For this review, take the finished solid that the model builds, in its own axes (mm). A direction names the side the tool comes from. Round coordinates to 2 decimals unless told otherwise and drop trailing zeros. Loops run counter-clockwise (first coordinate to the right, second up) from the corner with the lowest first, then second, coordinate; pieces in that order, holes last.
1. Draft analysis for pull direction Z (two halves, no side actions). For faces 1 (the cylindrical face through (2.958, 2.281, -123.594)), 2 (the flat face through (0, 91, -62)), 3 (the cylindrical face through (2.96, 44.25, -111.05)), state which applies: released by +Z, released by -Z, zero draft, split by the parting line, or undercut.
2. Tool access review of faces 4 (the cylindrical face through (2.96, 123.75, -38.91)), 5 (the flat face through (6, 91, -62)): name each direction out of +Z, -Z, +X, -X, +Y, -Y from which nothing blocks a thin tool from reaching the whole face with its end or side.
3. Consider section A-A on z = -111. State the section outline as (x, y) points, then the cut area to 3 significant figures.
4. Consider section B-B on y = 162.5. State the section outline as (x, z) points, then the cut area to 3 significant figures.
5. To check wall thickness, follow line 1 along Z through (x, y) = (5.35, 162); line 2 along Y through (x, z) = (4.45, -109); line 3 along Z through (x, y) = (3.2, 167.5). State the ranges of each line that lie inside material, in increasing order.
6. Consider section C-C on x = 1.5. State how many separate pieces and enclosed holes the cut face has, then the cut area to 3 significant figures.
from build123d import *

# Parameters (mm, degrees)
EXTRUDE_2_DEPTH          = 6
CUT_EXTRUDE_1_DEPTH      = 7
CUT_EXTRUDE_1_DEPTH_BACK = 1


with BuildPart() as part:
    # 草图1 → 凸台-拉伸2 (new body)
    with BuildSketch(Plane(origin=(0, 0, 0), x_dir=(0, 0, -1), z_dir=(1, 0, 0))):
        with BuildLine():
            Line((8, 0), (118, 0))
            ThreePointArc((118, 0), (123.656854249, 2.343145751), (126, 8))
            Line((126, 8), (126, 171.5))
            ThreePointArc((126, 171.5), (123.656854249, 177.156854249), (118, 179.5))
            Line((118, 179.5), (8, 179.5))
            ThreePointArc((8, 179.5), (2.343145751, 177.156854249), (0, 171.5))
            Line((0, 171.5), (0, 8))
            ThreePointArc((0, 8), (2.343145751, 2.343145751), (8, 0))
        make_face()
        with BuildLine():
            Line((12.75, 10), (12.75, 8))
            ThreePointArc((12.75, 8), (15, 5.75), (17.25, 8))
            Line((17.25, 8), (17.25, 10))
            ThreePointArc((17.25, 10), (15, 12.25), (12.75, 10))
        make_face(mode=Mode.SUBTRACT)
        with BuildLine():
            Line((12.75, 42), (12.75, 40))
            ThreePointArc((12.75, 40), (15, 37.75), (17.25, 40))
            Line((17.25, 40), (17.25, 42))
            ThreePointArc((17.25, 42), (15, 44.25), (12.75, 42))
        make_face(mode=Mode.SUBTRACT)
        with BuildLine():
            Line((108.75, 42), (108.75, 40))
            ThreePointArc((108.75, 40), (111, 37.75), (113.25, 40))
            Line((113.25, 40), (113.25, 42))
            ThreePointArc((113.25, 42), (111, 44.25), (108.75, 42))
        make_face(mode=Mode.SUBTRACT)
        with BuildLine():
            Line((108.75, 10), (108.75, 8))
            ThreePointArc((108.75, 8), (111, 5.75), (113.25, 8))
            Line((113.25, 8), (113.25, 10))
            ThreePointArc((113.25, 10), (111, 12.25), (108.75, 10))
        make_face(mode=Mode.SUBTRACT)
        with BuildLine():
            Line((60.75, 37.75), (63, 37.75))
            ThreePointArc((63, 37.75), (65.25, 40), (63, 42.25))
            Line((63, 42.25), (60.75, 42.25))
            ThreePointArc((60.75, 42.25), (58.5, 40), (60.75, 37.75))
        make_face(mode=Mode.SUBTRACT)
        with BuildLine():
            Line((60.75, 10.25), (63, 10.25))
            ThreePointArc((63, 10.25), (65.25, 8), (63, 5.75))
            Line((63, 5.75), (60.75, 5.75))
            ThreePointArc((60.75, 5.75), (58.5, 8), (60.75, 10.25))
        make_face(mode=Mode.SUBTRACT)
        with BuildLine():
            Line((34.75, 116.5), (34.75, 119.5))
            ThreePointArc((34.75, 119.5), (39, 123.75), (43.25, 119.5))
            Line((43.25, 119.5), (43.25, 116.5))
            ThreePointArc((43.25, 116.5), (39, 112.25), (34.75, 116.5))
        make_face(mode=Mode.SUBTRACT)
        with BuildLine():
            Line((82.75, 116.5), (82.75, 119.5))
            ThreePointArc((82.75, 119.5), (87, 123.75), (91.25, 119.5))
            Line((91.25, 119.5), (91.25, 116.5))
            ThreePointArc((91.25, 116.5), (87, 112.25), (82.75, 116.5))
        make_face(mode=Mode.SUBTRACT)
        with BuildLine():
            Line((10.75, 164.5), (10.75, 161.5))
            ThreePointArc((10.75, 161.5), (15, 157.25), (19.25, 161.5))
            Line((19.25, 161.5), (19.25, 164.5))
            ThreePointArc((19.25, 164.5), (15, 168.75), (10.75, 164.5))
        make_face(mode=Mode.SUBTRACT)
        with BuildLine():
            Line((67.25, 164.5), (67.25, 161.5))
            ThreePointArc((67.25, 161.5), (63, 157.25), (58.75, 161.5))
            Line((58.75, 161.5), (58.75, 164.5))
            ThreePointArc((58.75, 164.5), (63, 168.75), (67.25, 164.5))
        make_face(mode=Mode.SUBTRACT)
        with BuildLine():
            Line((115.25, 164.5), (115.25, 161.5))
            ThreePointArc((115.25, 161.5), (111, 157.25), (106.75, 161.5))
            Line((106.75, 161.5), (106.75, 164.5))
            ThreePointArc((106.75, 164.5), (111, 168.75), (115.25, 164.5))
        make_face(mode=Mode.SUBTRACT)
    extrude(amount=EXTRUDE_2_DEPTH)

    # 草图2 → 切除-拉伸1 (cut, two sides)
    with BuildSketch(Plane(origin=(0, 0, 0), x_dir=(0, 0, -1), z_dir=(1, 0, 0))) as cut_extrude_1_sk:
        with BuildLine():
            Line((43.25, 119.5), (43.25, 111.5))
            ThreePointArc((43.25, 111.5), (39, 107.25), (34.75, 111.5))
            Line((34.75, 111.5), (34.75, 119.5))
            ThreePointArc((34.75, 119.5), (39, 123.75), (43.25, 119.5))
        make_face()
        with BuildLine():
            Line((91.25, 119.5), (91.25, 111.5))
            ThreePointArc((91.25, 111.5), (87, 107.25), (82.75, 111.5))
            Line((82.75, 111.5), (82.75, 119.5))
            ThreePointArc((82.75, 119.5), (87, 123.75), (91.25, 119.5))
        make_face()
        with BuildLine():
            Line((19.25, 164.5), (19.25, 156.5))
            ThreePointArc((19.25, 156.5), (15, 152.25), (10.75, 156.5))
            Line((10.75, 156.5), (10.75, 164.5))
            ThreePointArc((10.75, 164.5), (15, 168.75), (19.25, 164.5))
        make_face()
        with BuildLine():
            Line((67.25, 164.5), (67.25, 156.5))
            ThreePointArc((67.25, 156.5), (63, 152.25), (58.75, 156.5))
            Line((58.75, 156.5), (58.75, 164.5))
            ThreePointArc((58.75, 164.5), (63, 168.75), (67.25, 164.5))
        make_face()
        with BuildLine():
            Line((115.25, 164.5), (115.25, 156.5))
            ThreePointArc((115.25, 156.5), (111, 152.25), (106.75, 156.5))
            Line((106.75, 156.5), (106.75, 164.5))
            ThreePointArc((106.75, 164.5), (111, 168.75), (115.25, 164.5))
        make_face()
    extrude(amount=CUT_EXTRUDE_1_DEPTH, mode=Mode.SUBTRACT)
    extrude(cut_extrude_1_sk.sketch, amount=-CUT_EXTRUDE_1_DEPTH_BACK, mode=Mode.SUBTRACT)


solid = part.part
Resolved:
1. face 1: released by -Z
1. face 2: zero draft
1. face 3: undercut
2. face 4: +X, -X
2. face 5: +Z, -Z, +X, +Y, -Y
3. outline: (0, 0) - (6, 0) - (6, 5.75) - (0, 5.75) - close; (0, 12.25) - (6, 12.25) - (6, 37.75) - (0, 37.75) - close; (0, 44.25) - (6, 44.25) - (6, 152.25) - (0, 152.25) - close; (0, 168.75) - (6, 168.75) - (6, 179.5) - (0, 179.5) - close
3. area: 900 mm2
4. outline: (0, -126) - (6, -126) - (6, -115.25) - (0, -115.25) - close; (0, -106.75) - (6, -106.75) - (6, -67.25) - (0, -67.25) - close; (0, -58.75) - (6, -58.75) - (6, -19.25) - (0, -19.25) - close; (0, -10.75) - (6, -10.75) - (6, 0) - (0, 0) - close
4. area: 603 mm2
5. line 1: z = -126 to -115.25, -106.75 to -67.25, -58.75 to -19.25, -10.75 to 0
5. line 2: y = 0 to 6.97, 11.03 to 38.97, 43.03 to 152.75, 168.25 to 179.5
5. line 3: z = -126 to -114.01, -107.99 to -66.01, -59.99 to -18.01, -11.99 to 0
6. separate pieces: 1
6. enclosed holes: 11
6. area: 21,800 mm2
